Here's how the part is built. I have some questions about the finished solid (model axes, mm). Face numbers are marked on the shaded views. Coordinates: 2 decimals unless noted, no trailing zeros. Loops run counter-clockwise (first coordinate to the right, second up) from the corner with the lowest first, then second, coordinate; pieces in that order, holes last. Notation, with made-up numbers: (64.5, 20) - (109.5, 20) arc R20 ccw to (109.5, 42) - close; hole circle Ø8 at (-12, 21.25). An arc over 180 degrees is marked (long way). Use a Markdown table: item, result.
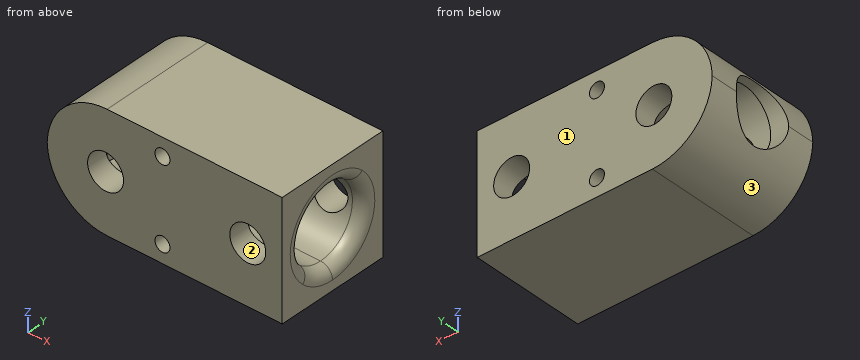
```python
from build123d import *

# Parameters (mm, degrees)
SKETCH1_W           = 39.25
SKETCH1_H           = 19.5
SKETCH1_R           = 1.25
SKETCH1_R_2         = 3
BOSS_EXTRUDE1_DEPTH = 19.25
CUT_EXTRUDE1_DEPTH  = 36.25
FILLET1_R           = 2
FILLET3_R           = 10
CUT_EXTRUDE3_REACH  = 47.441
SKETCH4_R           = 5


with BuildPart() as part:
    # Sketch1 → Boss-Extrude1 (new body)
    with BuildSketch(Plane(origin=(0, 0, 0), x_dir=(1, 0, 0), z_dir=(0, 1, 0))):
        with Locations((19.625, -9.75)):
            Rectangle(SKETCH1_W, SKETCH1_H)
        with Locations(Location((19.25, -16.5, 0), (0, 0, 270))):
            Circle(SKETCH1_R, mode=Mode.SUBTRACT)
        with Locations(Location((19.25, -3, 0), (0, 0, 270))):
            Circle(SKETCH1_R, mode=Mode.SUBTRACT)
        with Locations(Location((9.75, -9.75, 0), (0, 0, 270))):
            Circle(SKETCH1_R_2, mode=Mode.SUBTRACT)
        with Locations(Location((33.5, -9.75, 0), (0, 0, 270))):
            Circle(SKETCH1_R_2, mode=Mode.SUBTRACT)
    extrude(amount=BOSS_EXTRUDE1_DEPTH)

    # Sketch2 → Cut-Extrude1 (cut)
    with BuildSketch(Plane(origin=(39.25, 0, 0), x_dir=(0, 0, -1), z_dir=(1, 0, 0))):
        with BuildLine():
            ThreePointArc((-3.65, 9.625), (-7.433822489, 15.268165932), (-14.091089094, 13.910434106))
            Line((-14.091089094, 13.910434106), (-5.408910906, 5.339565894))
            ThreePointArc((-5.408910906, 5.339565894), (-4.106834068, 7.308822489), (-3.65, 9.625))
        make_face()
        with BuildLine():
            Line((-5.408910906, 5.339565894), (-14.091089094, 13.910434106))
            ThreePointArc((-14.091089094, 13.910434106), (-14.035434106, 5.283910906), (-5.408910906, 5.339565894))
        make_face()
    extrude(amount=-CUT_EXTRUDE1_DEPTH, mode=Mode.SUBTRACT)

    # Fillet1
    fillet1_edges = [part.edges().sort_by_distance(p)[0] for p in [
        (39.25, 5.339565894, 5.408910906),
    ]]
    fillet(fillet1_edges, radius=FILLET1_R)

    # Fillet3
    # the kernel refuses this fillet: 10 mm, written as the material it takes off along each edge
    with BuildSketch(Plane(origin=(0, -25, 19.5), x_dir=(1, 0, 0), z_dir=(0, 1, 0))) as fillet3_piece_1:
        with BuildLine():
            CenterArc((FILLET3_R, FILLET3_R), FILLET3_R, 180, 90)
            Line((0, FILLET3_R), (0, 0))
            Line((0, 0), (FILLET3_R, 0))
        make_face()
    extrude(amount=69.25, mode=Mode.SUBTRACT)
    with BuildSketch(Plane(origin=(0, -25, 0), x_dir=(1, 0, 0), z_dir=(0, 1, 0))) as fillet3_piece_2:
        with BuildLine():
            CenterArc((FILLET3_R, -FILLET3_R), FILLET3_R, 90, 90)
            Line((0, -FILLET3_R), (0, 0))
            Line((0, 0), (FILLET3_R, 0))
        make_face()
    extrude(amount=69.25, mode=Mode.SUBTRACT)

    # Sketch4 → Cut-Extrude3 (cut, up to next)
    with BuildSketch(Plane(origin=(3, 0, 0), x_dir=(0, 0, -1), z_dir=(1, 0, 0)), mode=Mode.PRIVATE) as cut_extrude3_sk1:
        with Locations((-9.75, 9.625)):
            Circle(SKETCH4_R)
    cut_extrude3_tool1 = extrude(cut_extrude3_sk1.sketch, amount=-CUT_EXTRUDE3_REACH, mode=Mode.PRIVATE) & part.part
    add(cut_extrude3_tool1.solids().sort_by_distance((3, 9.625, 9.75))[0], mode=Mode.SUBTRACT)


solid = part.part
```
Q1. Please list where these lines run through material, in increasing order: L1, parallel to X at y = 18.2, z = 9.75; L2, parallel to Z at x = 33.5, y = 3.3; L3, parallel to Y at x = 1.1, z = 9.75 (3 decimals). Write a range as from..to.
Check values:
| item | result |
|---|---|
| L1 | 0..6.75, 12.75..30.5, 36.5..39.25 |
| L2 | 0..6.75, 12.75..19.5 |
| L3 | 0..4.625, 14.625..19.25 |
Q2. If we mould it in two halves opening along Z, with no side actions, what happens to the marked faces 1, 2 and 3? For each: pulls with the +Z half, pulls with the -Z half, needs draft (parallel to the pull), parting line crosses it, or undercut.
Check values:
| item | result |
|---|---|
| face 1 | needs draft |
| face 2 | undercut |
| face 3 | pulls with the -Z half |
Q3. I want a section at B-B, the plane x = 19.25. Write out the boundary of the cut face in (y, z) (3 decimals), then the cut area to 3 significant figures.
Check values:
| item | result |
|---|---|
| outline | (0, 0) - (19.25, 0) - (19.25, 1.75) - (0, 1.75) - close; (0, 4.25) - (6.987, 4.25) arc R6.1 cw to (6.987, 15.25) - (0, 15.25) - close; (0, 17.75) - (19.25, 17.75) - (19.25, 19.5) - (0, 19.5) - close; (12.263, 4.25) - (19.25, 4.25) - (19.25, 15.25) - (12.263, 15.25) arc R6.1 cw to start |
| area | 166 mm^2 |
Q4. Will these pins go through, and if not, where does the flat tip stop? P1, Ø8, axis at x = 9.75, z = 9.75, coming from the +Y side; P2, Ø1, axis at y = 15.5, z = 6, coming from the +X side; P3, Ø10, axis at y = 7, z = 10, coming from the +X side; P4, Ø10, axis at y = 15.5, z = 17.5, coming from the -X side.
Check values:
| item | result |
|---|---|
| P1 | y = 19.25 |
| P2 | x = 39.15 |
| P3 | x = 39.2 |
| P4 | x = 0.46 |
Q5. I want a section at A-A, the plane x = 33.5. Write out the boundary of the cut face in (y, z) (3 decimals).
Check values:
| item | result |
|---|---|
| outline | (0, 0) - (19.25, 0) - (19.25, 6.75) - (14.936, 6.75) arc R6.1 cw to (4.314, 6.75) - (0, 6.75) - close; (0, 12.75) - (4.314, 12.75) arc R6.1 cw to (14.936, 12.75) - (19.25, 12.75) - (19.25, 19.5) - (0, 19.5) - close |
